Here's how the part is built. I have some questions about the finished solid (model axes, mm). Face numbers are marked on the shaded views. A direction names the side the tool comes from. Round coordinates to 2 decimals unless told otherwise and drop trailing zeros. Write each loop counter-clockwise with the first axis right and the second up, starting at its lowest first coordinate (ties: lowest second). Pieces come first, ordered by that corner, then holes. Notation, with made-up numbers: M -39.5,62 L 16.5,62 A32 ccw 16.5,95 Z; hole C 88,-38.5 d3. An arc over 180 degrees is marked long. Write item = value, one per line. Start each with the question number.
(1) On a 3-axis mill with a long thin cutter (end or side, diameter ignored), from which of +Z, -Z, +X, -X, +Y, -Y can I reach the whole of each face in a straight line? I mean the marked faces 4, 5, 6, 7 and 8. Say none if no direction works.
(2) I need wall thicknesses on line 1 along Y through (x, z) = (16.5, 0); line 2 along Y through (x, z) = (0, 20.8); line 3 along X through (y, z) = (5, -1.5). Which ranges of each line are inside material? Lowest first, please.
(3) I want a section at D-D (z = 10). List the corners of the cut face in (x, y) for me.
(4) If we mould it in two halves opening along Z, with no side actions, what happens to the marked faces 1, 2 and 3? For each: released by +Z, released by -Z, zero draft, split by the parting line, or undercut.
(5) Will these pins go through, and if not, where does the flat tip stop? pin 1 Ø1.5 at (x, z) = (5, 7.5) entering from -Y; pin 2 Ø2 at (x, y) = (-16.5, 15) entering from -Z; pin 3 Ø3 at (x, z) = (-17.5, 5.5) entering from -Y.
(6) I want a section at B-B (x = 16). List the corners of the cut face in (y, z) for me, and give its area (3 significant figures).
(7) I want a section at C-C (y = 15). List the corners of the cut face in (x, z) for me.
(8) I want a section at A-A (y = 5.5). List the corners of the cut face in (x, z) for me, and give its area (3 significant figures).
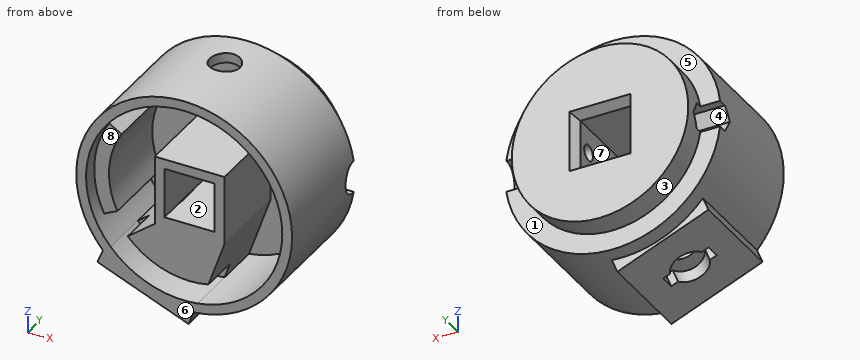
```python
from build123d import *
from OCP.BRepFilletAPI import BRepFilletAPI_MakeChamfer

# Parameters (mm, degrees)
SKETCH1_R                = 22
BOSS_EXTRUDE1_DEPTH      = 28
SKETCH2_W                = 10.2
SKETCH2_H                = 10.2
CUT_EXTRUDE2_DEPTH       = 42.856899073
SHELL3_T                 = -2
SKETCH3_R                = 3.1
CUT_EXTRUDE3_DEPTH       = 46.987063398
CHAMFER1_SIZE            = 2
CHAMFER1_SIZE2           = 1.154700538
BOSS_EXTRUDE8_START      = 23
BOSS_EXTRUDE8_DEPTH      = 23
BOSS_EXTRUDE4_DEPTH      = 20
BOSS_EXTRUDE6_DEPTH      = 26
CUT_EXTRUDE5_DEPTH       = 10
SKETCH13_R               = 3.8
CUT_EXTRUDE6_DEPTH       = 16
SKETCH15_W               = 10
SKETCH15_H               = 3
CUT_EXTRUDE8_DEPTH       = 16
CUT_EXTRUDE9_DEPTH       = 2
BOSS_EXTRUDE10_START     = 7
BOSS_EXTRUDE10_DEPTH     = 7
SKETCH21_OUTSIDE_W       = 60
SKETCH21_OUTSIDE_H       = 62.694
SKETCH21_OUTSIDE_R       = 18
CUT_EXTRUDE11_DEPTH      = 4.8
CUT_EXTRUDE12_DEPTH      = 47.132512216
CUT_EXTRUDE12_DEPTH_BACK = 47.132512216
SKETCH22_R               = 1.6
CUT_EXTRUDE13_START      = -8.5
SKETCH24_R               = 3.25
CUT_EXTRUDE13_DEPTH      = 38.632512277
CUT_EXTRUDE14_START      = -8.5
CUT_EXTRUDE14_DEPTH      = 38.632512278


with BuildPart() as part:
    # Sketch1 → Boss-Extrude1 (new body)
    with BuildSketch(Plane(origin=(0, 0, 0), x_dir=(1, 0, 0), z_dir=(0, 1, 0))):
        with Locations(Location((0, 0, 0), (0, 0, 270))):
            Circle(SKETCH1_R)
    extrude(amount=BOSS_EXTRUDE1_DEPTH)

    # Sketch2 → Cut-Extrude2 (cut, through all)
    with BuildSketch(Plane.XZ):
        Rectangle(SKETCH2_W, SKETCH2_H)
    extrude(amount=-CUT_EXTRUDE2_DEPTH, mode=Mode.SUBTRACT)

    # Shell3
    shell3_openings = [part.faces().sort_by_distance(p)[0] for p in [
        (0, 0, -21.377746033),
    ]]
    offset(amount=SHELL3_T, openings=shell3_openings, kind=Kind.INTERSECTION)

    # Sketch3 → Cut-Extrude3 (cut, through all)
    with BuildSketch(Plane.XY.offset(7.1)):
        with Locations(Location((0, 15, 0), (0, 0, 90.000000051))):
            Circle(SKETCH3_R)
    extrude(amount=CUT_EXTRUDE3_DEPTH, mode=Mode.SUBTRACT)

    # Chamfer1: one chamfer whose edges measure the first distance from different faces: ONE call of the kernel's chamfer builder (chamfer() names one face for all edges)
    chamfer1_edges_1 = [part.edges().sort_by_distance(p)[0] for p in [
        (5.1, 28, 0),
    ]]
    chamfer1_side_1 = [part.faces().sort_by_distance(p)[0] for p in [
        (5.1, 14, 0),
    ]]
    chamfer1_edges_2 = [part.edges().sort_by_distance(p)[0] for p in [
        (0, 28, -5.1),
    ]]
    chamfer1_side_2 = [part.faces().sort_by_distance(p)[0] for p in [
        (0, 14, -5.1),
    ]]
    chamfer1_edges_3 = [part.edges().sort_by_distance(p)[0] for p in [
        (-5.1, 28, 0),
    ]]
    chamfer1_side_3 = [part.faces().sort_by_distance(p)[0] for p in [
        (-5.1, 14, 0),
    ]]
    chamfer1_edges_4 = [part.edges().sort_by_distance(p)[0] for p in [
        (0, 28, 5.1),
    ]]
    chamfer1_side_4 = [part.faces().sort_by_distance(p)[0] for p in [
        (0, 14, 5.1),
    ]]
    chamfer1 = BRepFilletAPI_MakeChamfer(part.part.solid().wrapped)
    for e in chamfer1_edges_1:
        chamfer1.Add(CHAMFER1_SIZE, CHAMFER1_SIZE2, e.wrapped, chamfer1_side_1[0].wrapped)  # the first distance lies on this face
    for e in chamfer1_edges_2:
        chamfer1.Add(CHAMFER1_SIZE, CHAMFER1_SIZE2, e.wrapped, chamfer1_side_2[0].wrapped)  # the first distance lies on this face
    for e in chamfer1_edges_3:
        chamfer1.Add(CHAMFER1_SIZE, CHAMFER1_SIZE2, e.wrapped, chamfer1_side_3[0].wrapped)  # the first distance lies on this face
    for e in chamfer1_edges_4:
        chamfer1.Add(CHAMFER1_SIZE, CHAMFER1_SIZE2, e.wrapped, chamfer1_side_4[0].wrapped)  # the first distance lies on this face
    add(Compound.cast(chamfer1.Shape()), mode=Mode.REPLACE)

    # Sketch18 → Boss-Extrude8 (add)
    with BuildSketch(Plane.XZ.offset(-26).offset(BOSS_EXTRUDE8_START)):
        with BuildLine():
            Line((-15.279498787, -7.452309495), (-17.975880926, -8.767422936))
            ThreePointArc((-17.975880926, -8.767422936), (-19.972590695, 1.046719125), (-16.960961923, 10.598385285))
            Line((-16.960961923, 10.598385285), (-14.416817635, 9.008627492))
            ThreePointArc((-14.416817635, 9.008627492), (-16.976702091, 0.889711256), (-15.279498787, -7.452309495))
        make_face()
    extrude(amount=-BOSS_EXTRUDE8_DEPTH)

    # Sketch9 → Boss-Extrude4 (add)
    with BuildSketch(Plane.XZ):
        Polygon((1.996845621, -21.909190025), (-16.569234798, -14.472748814), (-17.684700979, -17.257660876), (0.881379439, -24.694102088), align=None)
    extrude(amount=-BOSS_EXTRUDE4_DEPTH)

    # Sketch11 → Boss-Extrude6 (add)
    with BuildSketch(Plane.XZ):
        with BuildLine():
            Line((1.996845621, -21.909190025), (7.1, -7.1))
            Line((7.1, -7.1), (-7.1, -7.1))
            Line((-7.1, -7.1), (-16.569234798, -14.472748814))
            ThreePointArc((-16.569234798, -14.472748814), (-8.180085333, -20.42268846), (1.996845621, -21.909190025))
        make_face()
    extrude(amount=-BOSS_EXTRUDE6_DEPTH)

    # Sketch12 → Cut-Extrude5 (cut)
    with BuildSketch(Plane.XZ):
        with BuildLine():
            Line((3.837309235, -16.568223759), (2.718713258, -19.814353338))
            ThreePointArc((2.718713258, -19.814353338), (-6.959564044, -18.750052488), (-14.988393562, -13.241905393))
            Line((-14.988393562, -13.241905393), (-12.621280739, -11.398870699))
            ThreePointArc((-12.621280739, -11.398870699), (-5.096085911, -16.225316302), (3.837309235, -16.568223759))
        make_face()
    extrude(amount=-CUT_EXTRUDE5_DEPTH, mode=Mode.SUBTRACT)

    # Sketch13 → Cut-Extrude6 (cut)
    with BuildSketch(Plane(origin=(-8.40166077, 0, -20.975881482), x_dir=(-0.9283040209233338, 0, 0.3718220605848592), z_dir=(-0.3718220605848592, 0, -0.9283040209233338))):
        with Locations((0, 10)):
            Circle(SKETCH13_R)
    extrude(amount=-CUT_EXTRUDE6_DEPTH, mode=Mode.SUBTRACT)

    # Sketch15 → Cut-Extrude8 (cut)
    with BuildSketch(Plane(origin=(-8.40166077, 0, -20.975881482), x_dir=(-0.9283040209233339, 0, 0.37182206058485906), z_dir=(-0.37182206058485906, 0, -0.9283040209233339))):
        with Locations((0, 10)):
            Rectangle(SKETCH15_W, SKETCH15_H)
    extrude(amount=-CUT_EXTRUDE8_DEPTH, mode=Mode.SUBTRACT)

    # Sketch17 → Cut-Extrude9 (cut)
    with BuildSketch(Plane.XZ):
        with BuildLine():
            Line((7.1, 7.1), (7.1, -7.1))
            Line((7.1, -7.1), (3.837309235, -16.568223759))
            ThreePointArc((3.837309235, -16.568223759), (-5.096085911, -16.225316302), (-12.621280739, -11.398870699))
            Line((-12.621280739, -11.398870699), (-7.1, -7.1))
            Line((-7.1, -7.1), (-7.1, 7.1))
            Line((-7.1, 7.1), (7.1, 7.1))
        make_face()
    extrude(amount=-CUT_EXTRUDE9_DEPTH, mode=Mode.SUBTRACT)

    # Sketch20 → Boss-Extrude10 (add)
    with BuildSketch(Plane.XZ.offset(-26).offset(BOSS_EXTRUDE10_START)):
        with BuildLine():
            Line((2.718713258, -19.814353338), (7.1, -7.1))
            Line((7.1, -7.1), (7.1, 7.1))
            Line((7.1, 7.1), (-7.1, 7.1))
            Line((-7.1, 7.1), (-7.1, -7.1))
            Line((-7.1, -7.1), (-14.988393562, -13.241905393))
            ThreePointArc((-14.988393562, -13.241905393), (6.959564044, 18.750052488), (2.718713258, -19.814353338))
        make_face()
    extrude(amount=-BOSS_EXTRUDE10_DEPTH)

    # Sketch21 outside → Cut-Extrude11 (cut)
    with BuildSketch(Plane(origin=(0, 28, 0), x_dir=(1, 0, 0), z_dir=(0, 1, 0))):
        with Locations((0, 1.347)):
            Rectangle(SKETCH21_OUTSIDE_W, SKETCH21_OUTSIDE_H)
        with Locations(Location((0, 0, 0), (0, 0, 270))):
            Circle(SKETCH21_OUTSIDE_R, mode=Mode.SUBTRACT)
    extrude(amount=-CUT_EXTRUDE11_DEPTH, mode=Mode.SUBTRACT)

    # Sketch22 → Cut-Extrude12 (cut, two sides: drawn at the far end of the back side and taken through both)
    with BuildSketch(Plane.ZY.offset(-5.1).offset(-CUT_EXTRUDE12_DEPTH_BACK)):
        with Locations((0, 23)):
            Circle(SKETCH22_R)
    extrude(amount=CUT_EXTRUDE12_DEPTH + CUT_EXTRUDE12_DEPTH_BACK, mode=Mode.SUBTRACT)

    # Sketch24 → Cut-Extrude13 (cut, through all)
    with BuildSketch(Plane.ZY.offset(-5.1).offset(CUT_EXTRUDE13_START)):
        with Locations((0, 23)):
            Circle(SKETCH24_R)
    extrude(amount=-CUT_EXTRUDE13_DEPTH, mode=Mode.SUBTRACT)

    # Sketch25 → Cut-Extrude14 (cut, through all)
    with BuildSketch(Plane(origin=(-5.1, 0, 0), x_dir=(0, 0, -1), z_dir=(1, 0, 0)).offset(CUT_EXTRUDE14_START)):
        Polygon((0, 19.893553151), (2.690261887, 21.446776575), (2.690261887, 24.553223425), (0, 26.106446849), (-2.690261887, 24.553223425), (-2.690261887, 21.446776575), align=None)
    extrude(amount=-CUT_EXTRUDE14_DEPTH, mode=Mode.SUBTRACT)


solid = part.part
```
Returned:
q1.face_4 = -X
q1.face_5 = +Z, +Y
q1.face_6 = +Z, -Z, +X, -X, -Y
q1.face_7 = +Y, -Y
q1.face_8 = -Y
q2.line_1 = 19 to 19.75, 26.25 to 28
q2.line_2 = 0 to 11.9, 18.1 to 23.2
q2.line_3 = -21.95 to -16.93, -7.1 to -5.1, 5.1 to 7.1, 19.94 to 21.95
q3.outline = M -19.6,0 L -17.32,0 L -17.32,3 L -16,3 L -16,19 L 17.32,19 L 17.32,0 L 19.6,0 L 19.6,23.2 L 14.97,23.2 L 14.97,28 L -14.97,28 L -14.97,23.2 L -19.6,23.2 Z
q4.face_1 = zero draft
q4.face_2 = undercut
q4.face_3 = split by the parting line
q5.pin_1 = 2
q5.pin_2 = -18.13
q5.pin_3 = 3
q6.outline = M 0,-15.1 L 23.2,-15.1 L 23.2,-8.25 L 28,-8.25 L 28,8.25 L 23.2,8.25 L 23.2,15.1 L 0,15.1 L 0,12 L 19,12 L 19,-12 L 0,-12 Z; hole C 23,0 d6.5
q6.area = 291 mm²
q7.outline = M -17.98,-8.77 L -15.28,-7.45 A17 cw -14.42,9.01 L -16.96,10.6 A20 cw -3.1,19.76 L -3.1,21.78 A22 ccw -16.57,-14.47 L -17.68,-17.26 L 0.88,-24.69 L 2,-21.91 A22 ccw 3.1,21.78 L 3.1,19.76 A20 cw 2.72,-19.81 L 7.1,-7.1 L 7.1,7.1 L -7.1,7.1 L -7.1,-7.1 L -14.99,-13.24 A20 cw Z; hole M -5.1,-5.1 L 5.1,-5.1 L 5.1,5.1 L -5.1,5.1 Z
q8.outline = M -17.68,-17.26 L 0.88,-24.69 L 2,-21.91 A22 ccw long -16.57,-14.47 Z; M -12.62,-11.4 A17.01 ccw 3.84,-16.57 L 7.1,-7.1 L 7.1,7.1 L -7.1,7.1 L -7.1,-7.1 Z; hole M -17.98,-8.77 A20 ccw long -16.96,10.6 L -14.42,9.01 A17 ccw -15.28,-7.45 Z; hole M -5.1,-5.1 L 5.1,-5.1 L 5.1,5.1 L -5.1,5.1 Z
q8.area = 590 mm²
